Autodesk Inventor part; units mm, degrees
ref_plane "YZ Plane" through (0, 0, 0) normal (1, 0, 0) x (0, 1, 0)
ref_plane "XZ Plane" through (0, 0, 0) normal (0, 1, 0) x (-1, 0, 0)
ref_plane "XY Plane" through (0, 0, 0) normal (0, 0, 1) x (1, 0, 0)
sketch "Sketch1" plane through (0, 0, 0) normal (0, 1, 0) x (-1, 0, 0)
  line L0 (0, 0) -> (25.4, 0)
  line L1 (25.4, 0) -> (25.4, -6.35)
  line L2 (25.4, -6.35) -> (0, -6.35)
  line L3 (0, -6.35) -> (0, 0)
  dimension "d0" = 25.4
  dimension "d1" = 6.35
extrude "Extrusion1" add sketch "Sketch1" along normal blind 3.175
sketch "Sketch2" plane through (0, 3.175, 0) normal (0, 1, 0) x (1, 0, 0)
  line L0 (0, 0) -> (0, 6.35)
  line L1 (0, 3.175) -> (-2.1082, 3.175)
  line L2 (-25.4, 6.35) -> (-25.4, 0)
  line L3 (-25.4, 3.175) -> (-23.2918, 3.175)
  dimension "d4" = 2.1082
  dimension "d5" = 2.1082
hole "Hole1" at (-23.2918, 3.175, -3.175) at (-2.1082, 3.175, -3.175) direction (0, -1, 0) diameter 3.2766 depth 5.6896 counterbore diameter 5.5626 counterbore depth 2.8448
fillet "Fillet1" radius 3.175 6 edges at (-12.7, 3.175, 0) (-12.7, 3.175, -6.35) (-25.4, 3.175, -5.6696) (-25.4, 3.175, -0.6804) (0, 3.175, -5.6696) (0, 3.175, -0.6804)
fillet "Fillet2" radius 3.175 4 edges at (0, 1.4698, -5.9893) (0, 1.4698, -0.3607) (-25.4, 1.4698, -5.9893) (-25.4, 1.4698, -0.3607)
properties part number "Retention Clip - Whisper Valve Horizontal"
Can you work these out from the model? Positions are in its coordinate system, mm. Coordinates: 2 decimals unless noted, no trailing zeros. Loops run counter-clockwise (first coordinate to the right, second up) from the corner with the lowest first, then second, coordinate; pieces in that order, holes last.
1) Imagine slicing it at D-D on y = 2.15. List the corners of the cut face in (x, z) for me (3 decimals), plus the area to 3 significant figures.
2) For pin 1 (3.5 mm diameter, centred on x = -2.11, z = -3.18, fed in from +Y), with a flat end and sliding along its axis, tell me the tip position at first contact or that it passes through.
3) Imagine slicing it at A-A on z = -2. List the corners of the cut face in (x, y) for me (3 decimals), plus the area to 3 significant figures.
4) I need wall thicknesses on probe 1 along Y at (x, z) = (-21.5, -2.75); probe 2 along X at (y, z) = (0.65, -5.25); probe 3 along Z at (x, y) = (-19.5, 2.4). Which ranges of each line are inside material? Lowest first, please.
5) Imagine slicing it at C-C on z = -3.5. List the corners of the cut face in (x, y) for me (3 decimals), plus the area to 3 significant figures.
6) Thinking about a two-plate mould opening in Z: for faces 1 (the cylindrical face through (-12.567, 3.174, -3.245)), 2 (the flat face through (-4, 0.33, -3)), 3 (the cylindrical face through (-1.48, 0.16, -1.66)), 4 (the flat face through (-13, 0, -3)), which applies, pulls with the +Z half, pulls with the -Z half, needs draft (parallel to the pull), parting line crosses it, or undercut?
7) Imagine slicing it at B-B on x = -18. List the corners of the cut face in (y, z) for me (3 decimals), plus the area to 3 significant figures.
Completed:
1. outline: (-21.783, -5.511) - (-3.617, -5.511) arc R2.781 cw to (-3.617, -0.839) - (-21.783, -0.839) arc R2.781 cw to start
1. area: 76.5 mm2
2. pin 1: stops at y = 0.33
3. outline: (-25.175, 0) - (-24.433, 0) - (-24.433, 0.33) - (-25.156, 0.33) arc R2.95 ccw to start; (-22.15, 0) - (-3.25, 0) - (-3.25, 0.33) - (-4.629, 0.33) - (-4.629, 2.95) - (-20.771, 2.95) - (-20.771, 0.33) - (-22.15, 0.33) - close; (-0.967, 0) - (-0.225, 0) arc R2.95 ccw to (-0.244, 0.33) - (-0.967, 0.33) - close
3. area: 49.0 mm2
4. probe 1: y = 0 to 0.33
4. probe 2: x = -21.44 to -3.96
4. probe 3: z = -5.25 to -1.1
5. outline: (-25.383, 0) - (-24.898, 0) - (-24.898, 0.33) - (-25.366, 0.33) arc R3.158 ccw to start; (-21.686, 0) - (-3.714, 0) - (-3.714, 0.33) - (-4.87, 0.33) - (-4.87, 3.158) - (-20.53, 3.158) - (-20.53, 0.33) - (-21.686, 0.33) - close; (-0.502, 0) - (-0.017, 0) arc R3.158 ccw to (-0.034, 0.33) - (-0.502, 0.33) - close
5. area: 50.5 mm2
6. face 1: parting line crosses it
6. face 2: undercut
6. face 3: undercut
6. face 4: needs draft
7. outline: (0, -6.35) arc R3.175 ccw to (0, 0) - close
7. area: 15.8 mm2
